Autodesk Inventor part; units mm, degrees
ref_plane "Work Plane1" through (-205, 2.4, 12.8522) normal (0, 1, 0) x (1, 0, 0)
ref_plane "Work Plane2" through (-205, 2.4, 12.8522) normal (0, 1, 0) x (1, 0, 0)
ref_plane "YZ Plane" through (0, 0, 0) normal (1, 0, 0) x (0, 1, 0)
ref_plane "Work Plane1" through (-205, 2.4, 12.8522) normal (0, 1, 0) x (1, 0, 0)
sketch "Sketch1" plane through (-205, 2.4, 12.8522) normal (0, 1, 0) x (1, 0, 0)
  line L0 (138.3655, -268.878) -> (91, -133.6728)
  line L1 (97.1039, -151.0965) -> (0, -93.5034)
  line L2 (0, 0) -> (0, -277.1478)
  circle A0 centre (132.5, -270.9328) radius 1.675
  circle A1 centre (132.5, -270.9328) radius 6.215
  line L3 (138.3655, -268.878) -> (97.1039, -151.0965)
  line L4 (132.5, -277.1478) -> (0, -277.1478)
  line L5 (0, -277.1478) -> (0, -93.5034)
  circle A2 centre (82.1326, -153.2062) radius 2.5
  circle A3 centre (82.1326, -153.2062) radius 2.5
  circle A4 centre (44.6303, -131.0762) radius 2.5
  circle A5 centre (44.6303, -131.0762) radius 2.5
  circle A6 centre (10.5733, -110.9794) radius 2.5
  circle A7 centre (10.5733, -110.9794) radius 2.5
  circle A8 centre (7.5, -154.9228) radius 1.675
  circle A9 centre (7.5, -154.9228) radius 1.675
  circle A10 centre (7.5, -270.9328) radius 1.675
  point P0 (205, 12.8522)
extrude "Extrusion1" add sketch "Sketch1" along normal blind 0.2
ref_plane "Work Plane2" through (-205, 2.4, 12.8522) normal (0, 1, 0) x (1, 0, 0)
sketch "Sketch2" plane through (-205, 2.4, 12.8522) normal (0, 1, 0) x (1, 0, 0)
  circle A0 centre (82.1326, -153.2062) radius 2.5
  circle A1 centre (82.1326, -153.2062) radius 2.5
  circle A2 centre (44.6303, -131.0762) radius 2.5
  circle A3 centre (44.6303, -131.0762) radius 2.5
  circle A4 centre (10.5733, -110.9794) radius 2.5
  circle A5 centre (10.5733, -110.9794) radius 2.5
  point P0 (205, 12.8522)
extrude "Extrusion2" add sketch "Sketch2" along normal blind 1
properties part number "base_main_pcb_p2_itr3"
Source: CAD feature listing. Evaluate the final solid. Frame: model axes, mm. A direction names the side the tool comes from. Round coordinates to 2 decimals unless told otherwise and drop trailing zeros. Loops run counter-clockwise (first coordinate to the right, second up) from the corner with the lowest first, then second, coordinate; pieces in that order, holes last.
(1) Contact query for flat-ended pins moving along their axis: pin 1 Ø2 at (x, z) = (-197.5, 283.785) entering from +Y; pin 2 Ø4.5 at (x, z) = (-72.5, 283.785) entering from +Y. Output: stop coordinate, or through.
From the geometry:
pin 1: passes through
pin 2: stops at y = 2.6
(2) Section query B-B (x = -101.5). Output: boundary loops of the cut face in (y, z), and give its area (3 significant figures).
From the geometry:
outline: (2.4, 182.21) - (2.6, 182.21) - (2.6, 290) - (2.4, 290) - close
area: 21.6 mm2
(3) Section query A-A (y = 3). Output: boundary loops of the cut face in (x, z), and give its area (3 significant figures).
From the geometry:
outline: circle Ø5 at (-194.43, 123.83); circle Ø5 at (-160.37, 143.93); circle Ø5 at (-122.87, 166.06)
area: 58.9 mm2
(4) Material intervals for probe 1 along Y at (x, z) = (-89, 269.5); probe 2 along Z at (x, y) = (-108, 2.55); probe 3 along X at (y, z) = (2.5, 177.5), sorted ascending.
From the geometry:
probe 1: y = 2.4 to 2.6
probe 2: z = 163.89 to 290
probe 3: x = -205 to -103.15
(5) Access query for faces 1 (the cylindrical face through (-121.523, 2.994, 168.166)), 2 (the flat face through (-152, 2.4, 217)). Directions: +Z, -Z, +X, -X, +Y, -Y. A direction counts if a zero-diameter tool reaches every point of the face in a straight line with its end or side. Return the directions, or none.
From the geometry:
face 1: +Y
face 2: +Z, -Z, +X, -X, -Y
